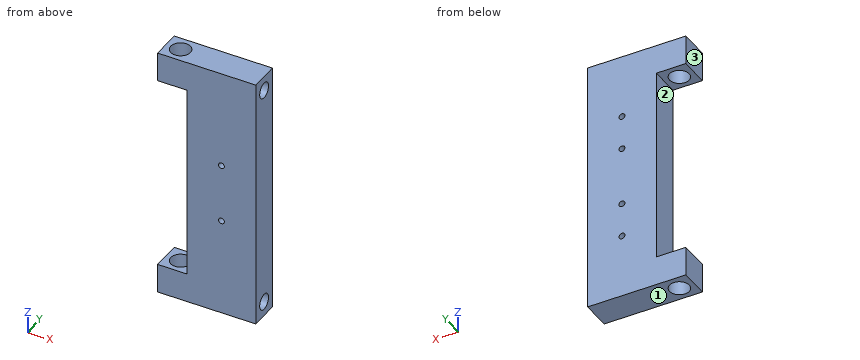
from build123d import *

# Parameters (mm, degrees)
ESQUISSE1_W             = 15
ESQUISSE1_H             = 15
ESQUISSE1_R             = 5
ESQUISSE1_W_2           = 35
BOSS_EXTRU_1_DEPTH      = 130
ESQUISSE2_W             = 15
ESQUISSE2_H             = 100
ENL_V_MAT_EXTRU_1_DEPTH = 60
ESQUISSE3_R             = 4
ENL_V_MAT_EXTRU_2_DEPTH = 35
ESQUISSE4_R             = 1.5
ENL_V_MAT_EXTRU_3_DEPTH = 5
ESQUISSE5_R             = 1.5
ENL_V_MAT_EXTRU_4_DEPTH = 15


with BuildPart() as part:
    # Esquisse1 → Boss.-Extru.1 (new body)
    with BuildSketch(Plane.XY):
        Rectangle(ESQUISSE1_W, ESQUISSE1_H)
        Circle(ESQUISSE1_R, mode=Mode.SUBTRACT)
        with Locations((25, 0)):
            Rectangle(ESQUISSE1_W_2, ESQUISSE1_H)
    extrude(amount=BOSS_EXTRU_1_DEPTH)

    # Esquisse2 → Enlèv. mat.-Extru.1 (cut)
    with BuildSketch(Plane(origin=(0, 7.5, 0), x_dir=(1, 0, 0), z_dir=(0, 1, 0))):
        with Locations((0, -65)):
            Rectangle(ESQUISSE2_W, ESQUISSE2_H)
    extrude(amount=-ENL_V_MAT_EXTRU_1_DEPTH, mode=Mode.SUBTRACT)

    # Esquisse3 → Enlèv. mat.-Extru.2 (cut)
    with BuildSketch(Plane(origin=(42.5, 0, 0), x_dir=(0, 0, -1), z_dir=(1, 0, 0))):
        with Locations((-122.5, 0)):
            Circle(ESQUISSE3_R)
        with Locations((-7.5, 0)):
            Circle(ESQUISSE3_R)
    extrude(amount=-ENL_V_MAT_EXTRU_2_DEPTH, mode=Mode.SUBTRACT)

    # Esquisse4 → Enlèv. mat.-Extru.3 (cut)
    with BuildSketch(Plane(origin=(0, 7.5, 0), x_dir=(1, 0, 0), z_dir=(0, 1, 0))):
        with Locations((25, -32.5)):
            Circle(ESQUISSE4_R)
        with Locations((25, -97.5)):
            Circle(ESQUISSE4_R)
    extrude(amount=-ENL_V_MAT_EXTRU_3_DEPTH, mode=Mode.SUBTRACT)

    # Esquisse5 → Enlèv. mat.-Extru.4 (cut)
    with BuildSketch(Plane(origin=(0, 7.5, 0), x_dir=(1, 0, 0), z_dir=(0, 1, 0))):
        with Locations((25, -50)):
            Circle(ESQUISSE5_R)
        with Locations((25, -80)):
            Circle(ESQUISSE5_R)
    extrude(amount=-ENL_V_MAT_EXTRU_4_DEPTH, mode=Mode.SUBTRACT)


solid = part.part
Source: CAD feature listing. Evaluate the final solid. Frame: model axes, mm. Face numbers are marked on the shaded views. Give positions to 0.01 mm unless a question says otherwise; leave off trailing zeros. Loops run counter-clockwise (first coordinate to the right, second up) from the corner with the lowest first, then second, coordinate; pieces in that order, holes last. Notation, with made-up numbers: (75.5, -9.5) -> (85.5, -9.5) arc R25 cw to (85.5, 7.5) -> close; hole circle Ø7 at (-33.75, 34.5). An arc over 180 degrees is marked (long way). Use a Markdown table: item, result. Add a question column.
1) Section query D-D, the plane y = -1.25. Return the cut outline in (x, z), then the cut area to 3 significant figures.
2) Section query C-C, the plane z = 122.5. Return the cut outline in (x, y), then the cut area to 3 significant figures.
3) Line query: line 1 along Z through (x, y) = (25, 6.2); line 2 along X through (y, z) = (0, 11.25); line 3 along Z through (x, y) = (4, -4). Output: solid intervals per line, ascending. Write a range as [from, to].
4) Section query A-A, the plane x = 25. Return the cut outline in (y, z), then the cut area to 3 significant figures.
5) First-contact query: pin 1 (4.5 mm diameter, centred on y = -1, z = 54.5, fed in from -X); pin 2 (7 mm diameter, centred on y = 0, z = 122.5, fed in from +X); pin 3 (2.5 mm diameter, centred on x = 25, z = 80, fed in from +Y); pin 4 (1.5 mm diameter, centred on x = 24.5, z = 32, fed in from +Y). Flat tips, straight axial feed; report the tip coordinate or a pass-through.
6) Section query B-B, the plane x = 0. Return the cut outline in (y, z).
7) Pull-direction query (Z, two-part tool) for the marked faces 1, 2 and 3; classes: +Z half, -Z half, draft (parallel to the pull), parting line (faces both ways), or undercut.
Numbers:
| question | item | result |
|---|---|---|
| 1 | outline | (-7.5, 0) -> (-4.84, 0) -> (-4.84, 15) -> (-7.5, 15) -> close; (-7.5, 115) -> (-4.84, 115) -> (-4.84, 130) -> (-7.5, 130) -> close; (4.84, 0) -> (42.5, 0) -> (42.5, 3.7) -> (7.5, 3.7) -> (7.5, 11.3) -> (42.5, 11.3) -> (42.5, 118.7) -> (7.5, 118.7) -> (7.5, 126.3) -> (42.5, 126.3) -> (42.5, 130) -> (4.84, 130) -> (4.84, 115) -> (7.5, 115) -> (7.5, 15) -> (4.84, 15) -> close; hole circle Ø3 at (25, 50); hole circle Ø3 at (25, 80) |
| 1 | area | 4,160 mm2 |
| 2 | outline | (-7.5, -7.5) -> (42.5, -7.5) -> (42.5, -4) -> (7.5, -4) -> (7.5, 4) -> (42.5, 4) -> (42.5, 7.5) -> (-7.5, 7.5) -> close; hole circle Ø10 at (0, 0) |
| 2 | area | 391 mm2 |
| 3 | line 1 | z = [0, 31], [34, 48.5], [51.5, 78.5], [81.5, 96], [99, 130] |
| 3 | line 2 | x = [-7.5, -5], [5, 7.5] |
| 3 | line 3 | z = [0, 15], [115, 130] |
| 4 | outline | (-7.5, 0) -> (7.5, 0) -> (7.5, 31) -> (2.5, 31) -> (2.5, 34) -> (7.5, 34) -> (7.5, 48.5) -> (-7.5, 48.5) -> close; (-7.5, 51.5) -> (7.5, 51.5) -> (7.5, 78.5) -> (-7.5, 78.5) -> close; (-7.5, 81.5) -> (7.5, 81.5) -> (7.5, 96) -> (2.5, 96) -> (2.5, 99) -> (7.5, 99) -> (7.5, 130) -> (-7.5, 130) -> close; hole circle Ø8 at (0, 7.5); hole circle Ø8 at (0, 122.5) |
| 4 | area | 1,730 mm2 |
| 5 | pin 1 | stops at x = 7.5 |
| 5 | pin 2 | stops at x = 7.5 |
| 5 | pin 3 | passes through |
| 5 | pin 4 | stops at y = 2.5 |
| 6 | outline | (-7.5, 0) -> (-5, 0) -> (-5, 15) -> (-7.5, 15) -> close; (-7.5, 115) -> (-5, 115) -> (-5, 130) -> (-7.5, 130) -> close; (5, 0) -> (7.5, 0) -> (7.5, 15) -> (5, 15) -> close; (5, 115) -> (7.5, 115) -> (7.5, 130) -> (5, 130) -> close |
| 7 | face 1 | -Z half |
| 7 | face 2 | undercut |
| 7 | face 3 | draft |
